Part model, mm, in its own coordinate system. Face numbers are marked on the shaded views. A direction names the side the tool comes from. Give positions to 0.01 mm unless a question says otherwise; leave off trailing zeros. Write each loop counter-clockwise with the first axis right and the second up, starting at its lowest first coordinate (ties: lowest second). Pieces come first, ordered by that corner, then holes.
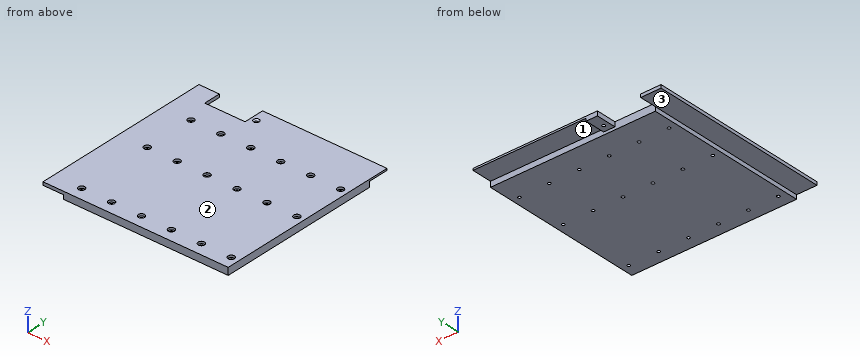
```python
from build123d import *

# Parameters (mm, degrees)
ESQUISSE1_W                                    = 408.5
ESQUISSE1_H                                    = 181
BOSS_EXTRU_1_DEPTH                             = 8
CHAMBRAGE_POUR_VIS_T_TE_RONDE_BOMB_2_COUNT     = 2
CHAMBRAGE_POUR_VIS_T_TE_RONDE_BOMB_2_PITCH     = 56
CHAMBRAGE_POUR_VIS_T_TE_RONDE_BOMB_3_COUNT     = 2
CHAMBRAGE_POUR_VIS_T_TE_RONDE_BOMB_3_PITCH     = 140
R_P_TITION_LIN_AIRE1_COUNT                     = 11
R_P_TITION_LIN_AIRE1_PITCH                     = 33
ENL_V_MAT_EXTRU_1_REACH                        = 275.026
ESQUISSE6_W                                    = 22.5
ESQUISSE6_H                                    = 4.5
BOSS_EXTRU_2_START                             = -3.5
ESQUISSE7_W                                    = 22.5
ESQUISSE7_H                                    = 18.725
BOSS_EXTRU_2_DEPTH                             = 3.5
ESQUISSE8_W                                    = 274.5
ESQUISSE8_H                                    = 22.375
BOSS_EXTRU_3_DEPTH                             = 5
FRAISAGE_POUR_VIS_T_TE_FRAIS_E_M31_D           = 3.4
FRAISAGE_POUR_VIS_T_TE_FRAIS_E_M31_CSINK_D     = 6.3
FRAISAGE_POUR_VIS_T_TE_FRAIS_E_M31_CSINK_ANGLE = 90
ESQUISSE12_W                                   = 249.5
ESQUISSE12_H                                   = 22.375
ENL_V_MAT_EXTRU_2_DEPTH                        = 3
ESQUISSE13_W                                   = 204.25
ESQUISSE13_H                                   = 203.375
ENL_V_MAT_EXTRU_3_DEPTH                        = 10


with BuildPart() as part:
    # Esquisse1 → Boss.-Extru.1 (new body)
    with BuildSketch(Plane.XY):
        Rectangle(ESQUISSE1_W, ESQUISSE1_H)
    extrude(amount=BOSS_EXTRU_1_DEPTH)

    # Esquisse3 → Chambrage pour vis à tête ronde bombée M31 (revolve, cut)
    with BuildSketch(Plane(origin=(-173.25, 63, 8), x_dir=(0, -1, 0), z_dir=(1, 0, 0))):
        Polygon((0, 0), (0, 8), (1.6, 8), (1.6, 2.4), (3.5, 2.4), (3.5, 0.025), (3.525, 0), align=None)
    chambrage_pour_vis_t_te_ronde_bomb_e_m = revolve(axis=Axis((-173.25, 63, 14.35), (0, 0, -1)), mode=Mode.SUBTRACT)

    # Chambrage pour vis _ t_te ronde bomb 2: Chambrage pour vis à tête ronde bombée M31 ×2
    with Locations(*[(0, -i * CHAMBRAGE_POUR_VIS_T_TE_RONDE_BOMB_2_PITCH, 0) for i in range(1, CHAMBRAGE_POUR_VIS_T_TE_RONDE_BOMB_2_COUNT)]):
        add(chambrage_pour_vis_t_te_ronde_bomb_e_m, mode=Mode.SUBTRACT)

    # Chambrage pour vis _ t_te ronde bomb 3: Chambrage pour vis à tête ronde bombée M31 ×2
    with Locations(*[(0, -i * CHAMBRAGE_POUR_VIS_T_TE_RONDE_BOMB_3_PITCH, 0) for i in range(1, CHAMBRAGE_POUR_VIS_T_TE_RONDE_BOMB_3_COUNT)]):
        add(chambrage_pour_vis_t_te_ronde_bomb_e_m, mode=Mode.SUBTRACT)

    # Répétition linéaire1: Chambrage pour vis à tête ronde bombée M31 ×11
    with Locations(*[(i * R_P_TITION_LIN_AIRE1_PITCH, 0, 0) for i in range(1, R_P_TITION_LIN_AIRE1_COUNT)]):
        add(chambrage_pour_vis_t_te_ronde_bomb_e_m, mode=Mode.SUBTRACT)

    # Répétition linéaire1 copy 1 sketch → Répétition linéaire1 copy 1 (revolve, cut)
    with BuildSketch(Plane(origin=(-140.25, 7, 8), x_dir=(0, -1, 0), z_dir=(1, 0, 0))):
        Polygon((0, 0), (0, 8), (1.6, 8), (1.6, 2.4), (3.5, 2.4), (3.5, 0.025), (3.525, 0), align=None)
    revolve(axis=Axis((-140.25, 7, 14.35), (0, 0, -1)), mode=Mode.SUBTRACT)

    # Répétition linéaire1 copy 2 sketch → Répétition linéaire1 copy 2 (revolve, cut)
    with BuildSketch(Plane(origin=(-107.25, 7, 8), x_dir=(0, -1, 0), z_dir=(1, 0, 0))):
        Polygon((0, 0), (0, 8), (1.6, 8), (1.6, 2.4), (3.5, 2.4), (3.5, 0.025), (3.525, 0), align=None)
    revolve(axis=Axis((-107.25, 7, 14.35), (0, 0, -1)), mode=Mode.SUBTRACT)

    # Répétition linéaire1 copy 3 sketch → Répétition linéaire1 copy 3 (revolve, cut)
    with BuildSketch(Plane(origin=(-74.25, 7, 8), x_dir=(0, -1, 0), z_dir=(1, 0, 0))):
        Polygon((0, 0), (0, 8), (1.6, 8), (1.6, 2.4), (3.5, 2.4), (3.5, 0.025), (3.525, 0), align=None)
    revolve(axis=Axis((-74.25, 7, 14.35), (0, 0, -1)), mode=Mode.SUBTRACT)

    # Répétition linéaire1 copy 4 sketch → Répétition linéaire1 copy 4 (revolve, cut)
    with BuildSketch(Plane(origin=(-41.25, 7, 8), x_dir=(0, -1, 0), z_dir=(1, 0, 0))):
        Polygon((0, 0), (0, 8), (1.6, 8), (1.6, 2.4), (3.5, 2.4), (3.5, 0.025), (3.525, 0), align=None)
    revolve(axis=Axis((-41.25, 7, 14.35), (0, 0, -1)), mode=Mode.SUBTRACT)

    # Répétition linéaire1 copy 5 sketch → Répétition linéaire1 copy 5 (revolve, cut)
    with BuildSketch(Plane(origin=(-8.25, 7, 8), x_dir=(0, -1, 0), z_dir=(1, 0, 0))):
        Polygon((0, 0), (0, 8), (1.6, 8), (1.6, 2.4), (3.5, 2.4), (3.5, 0.025), (3.525, 0), align=None)
    revolve(axis=Axis((-8.25, 7, 14.35), (0, 0, -1)), mode=Mode.SUBTRACT)

    # Répétition linéaire1 copy 6 sketch → Répétition linéaire1 copy 6 (revolve, cut)
    with BuildSketch(Plane(origin=(24.75, 7, 8), x_dir=(0, -1, 0), z_dir=(1, 0, 0))):
        Polygon((0, 0), (0, 8), (1.6, 8), (1.6, 2.4), (3.5, 2.4), (3.5, 0.025), (3.525, 0), align=None)
    revolve(axis=Axis((24.75, 7, 14.35), (0, 0, -1)), mode=Mode.SUBTRACT)

    # Répétition linéaire1 copy 7 sketch → Répétition linéaire1 copy 7 (revolve, cut)
    with BuildSketch(Plane(origin=(57.75, 7, 8), x_dir=(0, -1, 0), z_dir=(1, 0, 0))):
        Polygon((0, 0), (0, 8), (1.6, 8), (1.6, 2.4), (3.5, 2.4), (3.5, 0.025), (3.525, 0), align=None)
    revolve(axis=Axis((57.75, 7, 14.35), (0, 0, -1)), mode=Mode.SUBTRACT)

    # Répétition linéaire1 copy 8 sketch → Répétition linéaire1 copy 8 (revolve, cut)
    with BuildSketch(Plane(origin=(90.75, 7, 8), x_dir=(0, -1, 0), z_dir=(1, 0, 0))):
        Polygon((0, 0), (0, 8), (1.6, 8), (1.6, 2.4), (3.5, 2.4), (3.5, 0.025), (3.525, 0), align=None)
    revolve(axis=Axis((90.75, 7, 14.35), (0, 0, -1)), mode=Mode.SUBTRACT)

    # Répétition linéaire1 copy 9 sketch → Répétition linéaire1 copy 9 (revolve, cut)
    with BuildSketch(Plane(origin=(123.75, 7, 8), x_dir=(0, -1, 0), z_dir=(1, 0, 0))):
        Polygon((0, 0), (0, 8), (1.6, 8), (1.6, 2.4), (3.5, 2.4), (3.5, 0.025), (3.525, 0), align=None)
    revolve(axis=Axis((123.75, 7, 14.35), (0, 0, -1)), mode=Mode.SUBTRACT)

    # Répétition linéaire1 copy 10 sketch → Répétition linéaire1 copy 10 (revolve, cut)
    with BuildSketch(Plane(origin=(156.75, 7, 8), x_dir=(0, -1, 0), z_dir=(1, 0, 0))):
        Polygon((0, 0), (0, 8), (1.6, 8), (1.6, 2.4), (3.5, 2.4), (3.5, 0.025), (3.525, 0), align=None)
    revolve(axis=Axis((156.75, 7, 14.35), (0, 0, -1)), mode=Mode.SUBTRACT)

    # Répétition linéaire1 copy 11 sketch → Répétition linéaire1 copy 11 (revolve, cut)
    with BuildSketch(Plane(origin=(-140.25, -77, 8), x_dir=(0, -1, 0), z_dir=(1, 0, 0))):
        Polygon((0, 0), (0, 8), (1.6, 8), (1.6, 2.4), (3.5, 2.4), (3.5, 0.025), (3.525, 0), align=None)
    revolve(axis=Axis((-140.25, -77, 14.35), (0, 0, -1)), mode=Mode.SUBTRACT)

    # Répétition linéaire1 copy 12 sketch → Répétition linéaire1 copy 12 (revolve, cut)
    with BuildSketch(Plane(origin=(-107.25, -77, 8), x_dir=(0, -1, 0), z_dir=(1, 0, 0))):
        Polygon((0, 0), (0, 8), (1.6, 8), (1.6, 2.4), (3.5, 2.4), (3.5, 0.025), (3.525, 0), align=None)
    revolve(axis=Axis((-107.25, -77, 14.35), (0, 0, -1)), mode=Mode.SUBTRACT)

    # Répétition linéaire1 copy 13 sketch → Répétition linéaire1 copy 13 (revolve, cut)
    with BuildSketch(Plane(origin=(-74.25, -77, 8), x_dir=(0, -1, 0), z_dir=(1, 0, 0))):
        Polygon((0, 0), (0, 8), (1.6, 8), (1.6, 2.4), (3.5, 2.4), (3.5, 0.025), (3.525, 0), align=None)
    revolve(axis=Axis((-74.25, -77, 14.35), (0, 0, -1)), mode=Mode.SUBTRACT)

    # Répétition linéaire1 copy 14 sketch → Répétition linéaire1 copy 14 (revolve, cut)
    with BuildSketch(Plane(origin=(-41.25, -77, 8), x_dir=(0, -1, 0), z_dir=(1, 0, 0))):
        Polygon((0, 0), (0, 8), (1.6, 8), (1.6, 2.4), (3.5, 2.4), (3.5, 0.025), (3.525, 0), align=None)
    revolve(axis=Axis((-41.25, -77, 14.35), (0, 0, -1)), mode=Mode.SUBTRACT)

    # Répétition linéaire1 copy 15 sketch → Répétition linéaire1 copy 15 (revolve, cut)
    with BuildSketch(Plane(origin=(-8.25, -77, 8), x_dir=(0, -1, 0), z_dir=(1, 0, 0))):
        Polygon((0, 0), (0, 8), (1.6, 8), (1.6, 2.4), (3.5, 2.4), (3.5, 0.025), (3.525, 0), align=None)
    revolve(axis=Axis((-8.25, -77, 14.35), (0, 0, -1)), mode=Mode.SUBTRACT)

    # Répétition linéaire1 copy 16 sketch → Répétition linéaire1 copy 16 (revolve, cut)
    with BuildSketch(Plane(origin=(24.75, -77, 8), x_dir=(0, -1, 0), z_dir=(1, 0, 0))):
        Polygon((0, 0), (0, 8), (1.6, 8), (1.6, 2.4), (3.5, 2.4), (3.5, 0.025), (3.525, 0), align=None)
    revolve(axis=Axis((24.75, -77, 14.35), (0, 0, -1)), mode=Mode.SUBTRACT)

    # Répétition linéaire1 copy 17 sketch → Répétition linéaire1 copy 17 (revolve, cut)
    with BuildSketch(Plane(origin=(57.75, -77, 8), x_dir=(0, -1, 0), z_dir=(1, 0, 0))):
        Polygon((0, 0), (0, 8), (1.6, 8), (1.6, 2.4), (3.5, 2.4), (3.5, 0.025), (3.525, 0), align=None)
    revolve(axis=Axis((57.75, -77, 14.35), (0, 0, -1)), mode=Mode.SUBTRACT)

    # Répétition linéaire1 copy 18 sketch → Répétition linéaire1 copy 18 (revolve, cut)
    with BuildSketch(Plane(origin=(90.75, -77, 8), x_dir=(0, -1, 0), z_dir=(1, 0, 0))):
        Polygon((0, 0), (0, 8), (1.6, 8), (1.6, 2.4), (3.5, 2.4), (3.5, 0.025), (3.525, 0), align=None)
    revolve(axis=Axis((90.75, -77, 14.35), (0, 0, -1)), mode=Mode.SUBTRACT)

    # Répétition linéaire1 copy 19 sketch → Répétition linéaire1 copy 19 (revolve, cut)
    with BuildSketch(Plane(origin=(123.75, -77, 8), x_dir=(0, -1, 0), z_dir=(1, 0, 0))):
        Polygon((0, 0), (0, 8), (1.6, 8), (1.6, 2.4), (3.5, 2.4), (3.5, 0.025), (3.525, 0), align=None)
    revolve(axis=Axis((123.75, -77, 14.35), (0, 0, -1)), mode=Mode.SUBTRACT)

    # Répétition linéaire1 copy 20 sketch → Répétition linéaire1 copy 20 (revolve, cut)
    with BuildSketch(Plane(origin=(156.75, -77, 8), x_dir=(0, -1, 0), z_dir=(1, 0, 0))):
        Polygon((0, 0), (0, 8), (1.6, 8), (1.6, 2.4), (3.5, 2.4), (3.5, 0.025), (3.525, 0), align=None)
    revolve(axis=Axis((156.75, -77, 14.35), (0, 0, -1)), mode=Mode.SUBTRACT)

    # Esquisse6 → Enlèv. mat.-Extru.1 (cut, up to next)
    with BuildSketch(Plane(origin=(0, 90.5, 0), x_dir=(1, 0, 0), z_dir=(0, 1, 0)), mode=Mode.PRIVATE) as enl_v_mat_extru_1_sk1:
        with Locations((-193, -2.25)):
            Rectangle(ESQUISSE6_W, ESQUISSE6_H)
    enl_v_mat_extru_1_tool1 = extrude(enl_v_mat_extru_1_sk1.sketch, amount=-ENL_V_MAT_EXTRU_1_REACH, mode=Mode.PRIVATE) & part.part
    # Esquisse6 → Enlèv. mat.-Extru.1 (cut, up to next)
    with BuildSketch(Plane(origin=(0, 90.5, 0), x_dir=(1, 0, 0), z_dir=(0, 1, 0)), mode=Mode.PRIVATE) as enl_v_mat_extru_1_sk2:
        with Locations((193, -2.25)):
            Rectangle(ESQUISSE6_W, ESQUISSE6_H)
    enl_v_mat_extru_1_tool2 = extrude(enl_v_mat_extru_1_sk2.sketch, amount=-ENL_V_MAT_EXTRU_1_REACH, mode=Mode.PRIVATE) & part.part
    add(enl_v_mat_extru_1_tool1.solids().sort_by_distance((-193, 90.5, 2.25))[0], mode=Mode.SUBTRACT)
    add(enl_v_mat_extru_1_tool2.solids().sort_by_distance((193, 90.5, 2.25))[0], mode=Mode.SUBTRACT)

    # Esquisse7 → Boss.-Extru.2 (add)
    with BuildSketch(Plane.XY.offset(8).offset(BOSS_EXTRU_2_START)):
        with Locations((-193, 99.8625)):
            Rectangle(ESQUISSE7_W, ESQUISSE7_H)
    boss_extru_2 = extrude(amount=BOSS_EXTRU_2_DEPTH)

    # Symétrie1: Boss.-Extru.2 across plane
    add(boss_extru_2.mirror(Plane(origin=(0, 0, 0), x_dir=(0, 0, 1), z_dir=(1, 0, 0))))

    # Esquisse8 → Boss.-Extru.3 (add)
    with BuildSketch(Plane.XY.offset(8)):
        with Locations((0, 101.6875)):
            Rectangle(ESQUISSE8_W, ESQUISSE8_H)
    extrude(amount=-BOSS_EXTRU_3_DEPTH)

    # Fraisage pour vis à tête fraisée M31 (through all)
    with Locations(Plane.XY.offset(8)):
        with Locations((-131.25, 98), (131.25, 98)):
            CounterSinkHole(FRAISAGE_POUR_VIS_T_TE_FRAIS_E_M31_D / 2, FRAISAGE_POUR_VIS_T_TE_FRAIS_E_M31_CSINK_D / 2, counter_sink_angle=FRAISAGE_POUR_VIS_T_TE_FRAIS_E_M31_CSINK_ANGLE)

    # Esquisse12 → Enlèv. mat.-Extru.2 (cut)
    with BuildSketch(Plane(origin=(0, 0, 3), x_dir=(-1, 0, 0), z_dir=(0, 0, -1))):
        with Locations((0, 101.6875)):
            Rectangle(ESQUISSE12_W, ESQUISSE12_H)
    extrude(amount=-ENL_V_MAT_EXTRU_2_DEPTH, mode=Mode.SUBTRACT)

    # Esquisse13 → Enlèv. mat.-Extru.3 (cut)
    with BuildSketch(Plane(origin=(0, 0, 0), x_dir=(-1, 0, 0), z_dir=(0, 0, -1))):
        with Locations((-102.125, 11.1875)):
            Rectangle(ESQUISSE13_W, ESQUISSE13_H)
    extrude(amount=-ENL_V_MAT_EXTRU_3_DEPTH, mode=Mode.SUBTRACT)


solid = part.part
```
1) 3-axis set-ups, long thin cutter, end or side, ignore diameter. For the marked faces 1, 2 and 3: which of +Z, -Z, +X, -X, +Y, -Y reach the whole face in a straight line?
Answers follow:
face 1: -Z, +X, +Y
face 2: +Z, +X, -X, +Y, -Y
face 3: -Z, -X, +Y, -Y
2) Wall check: L1, parallel to Y at x = -74.25, z = 3.35; L2, parallel to X at y = 98, z = 5; L3, parallel to Y at x = -75.5, z = 1.75. Give the ranges that are in metal, low to high.
Answers follow:
L1: y = -90.5 to -78.6, -75.4 to 5.4, 8.6 to 61.4, 64.6 to 90.5
L2: x = -204.25 to -181.75, -137.25 to -132.95, -129.55 to -124.75
L3: y = -90.5 to -78, -76 to 6, 8 to 62, 64 to 90.5
3) Saw through at A-A, the plane y = -32.5. Write the cut outline in (x, z).
Answers follow:
outline: (-204.25, 4.5) - (-181.75, 4.5) - (-181.75, 0) - (0, 0) - (0, 8) - (-204.25, 8) - close
4) Pin check, flat tips, straight feed: pin 1 Ø4 at (x, y) = (-107.25, -77) entering from +Z; pin 2 Ø2.5 at (y, z) = (106.5, 4.5) entering from +X; pin 3 Ø1.3 at (y, z) = (-33, 1.5) entering from -X; pin 4 Ø2.5 at (x, y) = (-173.25, -77) entering from +Z (3 decimals). Stop position of each tip, or through.
Answers follow:
pin 1: stops at z = 5.6
pin 2: stops at x = -124.75
pin 3: stops at x = -181.75
pin 4: passes through
5) Saw through at C-C, the plane x = -186. Write the cut outline in (y, z) (3 decimals).
Answers follow:
outline: (-90.5, 4.5) - (109.225, 4.5) - (109.225, 8) - (-90.5, 8) - close
6) Saw through at B-B, the plane x = -33.5. Write the cut outline in (y, z) (3 decimals), then the cut area to 3 significant figures.
Answers follow:
outline: (-90.5, 0) - (90.5, 0) - (90.5, 6) - (112.875, 6) - (112.875, 8) - (-90.5, 8) - close
area: 1,490 mm2
